Work out the finished part from the listing and answer in its coordinate system (mm). Face numbers are marked on the shaded views. A direction names the side the tool comes from. Round coordinates to 2 decimals unless told otherwise and drop trailing zeros. Write each loop counter-clockwise with the first axis right and the second up, starting at its lowest first coordinate (ties: lowest second). Pieces come first, ordered by that corner, then holes. Notation, with made-up numbers: M -23.5,78.25 L 10.5,78.25 A7 ccw 10.5,86.25 Z; hole C -25,-34 d4. An arc over 180 degrees is marked long. Answer in a Markdown table with one row per item.
```python
from build123d import *

# Parameters (mm, degrees)
SKETCH1_R           = 7.95
SKETCH1_R_2         = 2.3
BOSS_EXTRUDE1_DEPTH = 7.3
SKETCH2_R           = 2.3
BOSS_EXTRUDE2_DEPTH = 6.8
SKETCH3_R           = 7.95
SKETCH3_R_2         = 2.3
BOSS_EXTRUDE3_DEPTH = 1.3
CHAMFER1_SIZE       = 0.3


with BuildPart() as part:
    # Sketch1 → Boss-Extrude1 (new body)
    with BuildSketch(Plane(origin=(0, 0, 0), x_dir=(1, 0, 0), z_dir=(0, 1, 0))):
        with Locations(Location((0, 0, 0), (0, 0, 270))):
            Circle(SKETCH1_R)
        with Locations(Location((0, 0, 0), (0, 0, 270))):
            Circle(SKETCH1_R_2, mode=Mode.SUBTRACT)
    extrude(amount=BOSS_EXTRUDE1_DEPTH)

    # Sketch2 → Boss-Extrude2 (add)
    with BuildSketch(Plane(origin=(0, 7.3, 0), x_dir=(1, 0, 0), z_dir=(0, 1, 0))):
        with BuildLine():
            Line((1.565184181, 6.273372178), (1.420904518, 5.829325034))
            ThreePointArc((1.420904518, 5.829325034), (0.93860679, 5.926130044), (0.45, 5.983101203))
            Line((0.45, 5.983101203), (0.45, 6.45))
            Line((0.45, 6.45), (-0.45, 6.45))
            Line((-0.45, 6.45), (-0.45, 5.983101203))
            ThreePointArc((-0.45, 5.983101203), (-0.93860679, 5.926130044), (-1.420904518, 5.829325034))
            Line((-1.420904518, 5.829325034), (-1.565184181, 6.273372178))
            Line((-1.565184181, 6.273372178), (-2.421135046, 5.995256883))
            Line((-2.421135046, 5.995256883), (-2.276855383, 5.551209739))
            ThreePointArc((-2.276855383, 5.551209739), (-2.723942998, 5.346039145), (-3.152721002, 5.104933915))
            Line((-3.152721002, 5.104933915), (-3.42715723, 5.482662977))
            Line((-3.42715723, 5.482662977), (-4.155272525, 4.95365625))
            Line((-4.155272525, 4.95365625), (-3.880836297, 4.575927188))
            ThreePointArc((-3.880836297, 4.575927188), (-4.242640687, 4.242640687), (-4.575927188, 3.880836297))
            Line((-4.575927188, 3.880836297), (-4.95365625, 4.155272525))
            Line((-4.95365625, 4.155272525), (-5.482662977, 3.42715723))
            Line((-5.482662977, 3.42715723), (-5.104933915, 3.152721002))
            ThreePointArc((-5.104933915, 3.152721002), (-5.346039145, 2.723942998), (-5.551209739, 2.276855383))
            Line((-5.551209739, 2.276855383), (-5.995256883, 2.421135046))
            Line((-5.995256883, 2.421135046), (-6.273372178, 1.565184181))
            Line((-6.273372178, 1.565184181), (-5.829325034, 1.420904518))
            ThreePointArc((-5.829325034, 1.420904518), (-5.926130044, 0.93860679), (-5.983101203, 0.45))
            Line((-5.983101203, 0.45), (-6.45, 0.45))
            Line((-6.45, 0.45), (-6.45, -0.45))
            Line((-6.45, -0.45), (-5.983101203, -0.45))
            ThreePointArc((-5.983101203, -0.45), (-5.926130044, -0.93860679), (-5.829325034, -1.420904518))
            Line((-5.829325034, -1.420904518), (-6.273372178, -1.565184181))
            Line((-6.273372178, -1.565184181), (-5.995256883, -2.421135046))
            Line((-5.995256883, -2.421135046), (-5.551209739, -2.276855383))
            ThreePointArc((-5.551209739, -2.276855383), (-5.346039145, -2.723942998), (-5.104933915, -3.152721002))
            Line((-5.104933915, -3.152721002), (-5.482662977, -3.42715723))
            Line((-5.482662977, -3.42715723), (-4.95365625, -4.155272525))
            Line((-4.95365625, -4.155272525), (-4.575927188, -3.880836297))
            ThreePointArc((-4.575927188, -3.880836297), (-4.242640687, -4.242640687), (-3.880836297, -4.575927188))
            Line((-3.880836297, -4.575927188), (-4.155272525, -4.95365625))
            Line((-4.155272525, -4.95365625), (-3.42715723, -5.482662977))
            Line((-3.42715723, -5.482662977), (-3.152721002, -5.104933915))
            ThreePointArc((-3.152721002, -5.104933915), (-2.723942998, -5.346039145), (-2.276855383, -5.551209739))
            Line((-2.276855383, -5.551209739), (-2.421135046, -5.995256883))
            Line((-2.421135046, -5.995256883), (-1.565184181, -6.273372178))
            Line((-1.565184181, -6.273372178), (-1.420904518, -5.829325034))
            ThreePointArc((-1.420904518, -5.829325034), (-0.93860679, -5.926130044), (-0.45, -5.983101203))
            Line((-0.45, -5.983101203), (-0.45, -6.45))
            Line((-0.45, -6.45), (0.45, -6.45))
            Line((0.45, -6.45), (0.45, -5.983101203))
            ThreePointArc((0.45, -5.983101203), (0.93860679, -5.926130044), (1.420904518, -5.829325034))
            Line((1.420904518, -5.829325034), (1.565184181, -6.273372178))
            Line((1.565184181, -6.273372178), (2.421135046, -5.995256883))
            Line((2.421135046, -5.995256883), (2.276855383, -5.551209739))
            ThreePointArc((2.276855383, -5.551209739), (2.723942998, -5.346039145), (3.152721002, -5.104933915))
            Line((3.152721002, -5.104933915), (3.42715723, -5.482662977))
            Line((3.42715723, -5.482662977), (4.155272525, -4.95365625))
            Line((4.155272525, -4.95365625), (3.880836297, -4.575927188))
            ThreePointArc((3.880836297, -4.575927188), (4.242640687, -4.242640687), (4.575927188, -3.880836297))
            Line((4.575927188, -3.880836297), (4.95365625, -4.155272525))
            Line((4.95365625, -4.155272525), (5.482662977, -3.42715723))
            Line((5.482662977, -3.42715723), (5.104933915, -3.152721002))
            ThreePointArc((5.104933915, -3.152721002), (5.346039145, -2.723942998), (5.551209739, -2.276855383))
            Line((5.551209739, -2.276855383), (5.995256883, -2.421135046))
            Line((5.995256883, -2.421135046), (6.273372178, -1.565184181))
            Line((6.273372178, -1.565184181), (5.829325034, -1.420904518))
            ThreePointArc((5.829325034, -1.420904518), (5.926130044, -0.93860679), (5.983101203, -0.45))
            Line((5.983101203, -0.45), (6.45, -0.45))
            Line((6.45, -0.45), (6.45, 0.45))
            Line((6.45, 0.45), (5.983101203, 0.45))
            ThreePointArc((5.983101203, 0.45), (5.926130044, 0.93860679), (5.829325034, 1.420904518))
            Line((5.829325034, 1.420904518), (6.273372178, 1.565184181))
            Line((6.273372178, 1.565184181), (5.995256883, 2.421135046))
            Line((5.995256883, 2.421135046), (5.551209739, 2.276855383))
            ThreePointArc((5.551209739, 2.276855383), (5.346039145, 2.723942998), (5.104933915, 3.152721002))
            Line((5.104933915, 3.152721002), (5.482662977, 3.42715723))
            Line((5.482662977, 3.42715723), (4.95365625, 4.155272525))
            Line((4.95365625, 4.155272525), (4.575927188, 3.880836297))
            ThreePointArc((4.575927188, 3.880836297), (4.242640687, 4.242640687), (3.880836297, 4.575927188))
            Line((3.880836297, 4.575927188), (4.155272525, 4.95365625))
            Line((4.155272525, 4.95365625), (3.42715723, 5.482662977))
            Line((3.42715723, 5.482662977), (3.152721002, 5.104933915))
            ThreePointArc((3.152721002, 5.104933915), (2.723942998, 5.346039145), (2.276855383, 5.551209739))
            Line((2.276855383, 5.551209739), (2.421135046, 5.995256883))
            Line((2.421135046, 5.995256883), (1.565184181, 6.273372178))
        make_face()
        with Locations(Location((0, 0, 0), (0, 0, 270))):
            Circle(SKETCH2_R, mode=Mode.SUBTRACT)
    extrude(amount=BOSS_EXTRUDE2_DEPTH)

    # Sketch3 → Boss-Extrude3 (add)
    with BuildSketch(Plane(origin=(0, 14.1, 0), x_dir=(1, 0, 0), z_dir=(0, 1, 0))):
        with Locations(Location((0, 0, 0), (0, 0, 270))):
            Circle(SKETCH3_R)
        with Locations(Location((0, 0, 0), (0, 0, 270))):
            Circle(SKETCH3_R_2, mode=Mode.SUBTRACT)
    extrude(amount=BOSS_EXTRUDE3_DEPTH)

    # Chamfer1
    chamfer1_edges = [part.edges().sort_by_distance(p)[0] for p in [
        (0, 0, -7.95),
        (0, 15.4, -7.95),
        (0, 14.1, -7.95),
        (0, 7.3, -7.95),
    ]]
    chamfer(chamfer1_edges, length=CHAMFER1_SIZE)


solid = part.part
```
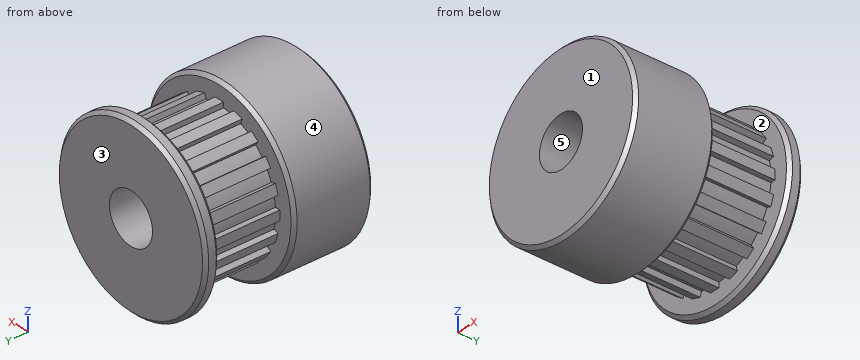
1. A tool of negligible diameter and unlimited length cuts with its end or side. For the marked faces 1 and 2, from which of +Z, -Z, +X, -X, +Y, -Y can it reach the whole face along a straight path? Write none if from no direction.
Calculated:
| item | result |
|---|---|
| face 1 | +Z, -Z, +X, -X, -Y |
| face 2 | none |
2. The part is cut by section C-C (y = 6.5). Determine the outline of the cut face in (x, z), plus the area to 3 significant figures.
Calculated:
| item | result |
|---|---|
| outline | C 0,0 d15.9; hole C 0,0 d4.6 |
| area | 182 mm² |
3. Consider line 1 along X through (y, z) = (9.5, 0); line 2 along Y through (x, z) = (7, -2.5); line 3 along X through (y, z) = (6.5, 0). Determine where each line is inside the solid, lowest interval first. Write a range as from..to.
Calculated:
| item | result |
|---|---|
| line 1 | x = -6.45..-2.3, 2.3..6.45 |
| line 2 | y = 0..7.3, 14.1..15.4 |
| line 3 | x = -7.95..-2.3, 2.3..7.95 |
4. The part is cut by section A-A (z = 0). Determine the outline of the cut face in (x, y), plus the area to 3 significant figures.
Calculated:
| item | result |
|---|---|
| outline | M -7.95,0.3 L -7.65,0 L -2.3,0 L -2.3,15.4 L -7.65,15.4 L -7.95,15.1 L -7.95,14.4 L -7.65,14.1 L -6.45,14.1 L -6.45,7.3 L -7.65,7.3 L -7.95,7 Z; M 2.3,0 L 7.65,0 L 7.95,0.3 L 7.95,7 L 7.65,7.3 L 6.45,7.3 L 6.45,14.1 L 7.65,14.1 L 7.95,14.4 L 7.95,15.1 L 7.65,15.4 L 2.3,15.4 Z |
| area | 153 mm² |
5. The part is cut by section B-B (x = 0). Determine the outline of the cut face in (y, z).
Calculated:
| item | result |
|---|---|
| outline | M 0,-7.65 L 0.3,-7.95 L 7,-7.95 L 7.3,-7.65 L 7.3,-6.45 L 14.1,-6.45 L 14.1,-7.65 L 14.4,-7.95 L 15.1,-7.95 L 15.4,-7.65 L 15.4,-2.3 L 0,-2.3 Z; M 0,2.3 L 15.4,2.3 L 15.4,7.65 L 15.1,7.95 L 14.4,7.95 L 14.1,7.65 L 14.1,6.45 L 7.3,6.45 L 7.3,7.65 L 7,7.95 L 0.3,7.95 L 0,7.65 Z |
6. Given pin 1 (0.5 mm diameter, centred on y = 12, z = -6, fed in from -X); pin 2 (0.5 mm diameter, centred on x = 6, y = 10.5, fed in from +Z); pin 3 (0.5 mm diameter, centred on x = -6, y = 11, fed in from -Z), each flat-ended and moving along its own axis, determine where each tip first touches the part or whether it passes through.
Calculated:
| item | result |
|---|---|
| pin 1 | stops at x = -2.42 |
| pin 2 | stops at z = 2.42 |
| pin 3 | stops at z = -2.42 |
7. Determine the mould class of the marked faces 3, 4 and 5 for opening direction X: released by +X, released by -X, zero draft, split by the parting line, or undercut.
Calculated:
| item | result |
|---|---|
| face 3 | zero draft |
| face 4 | split by the parting line |
| face 5 | undercut |
